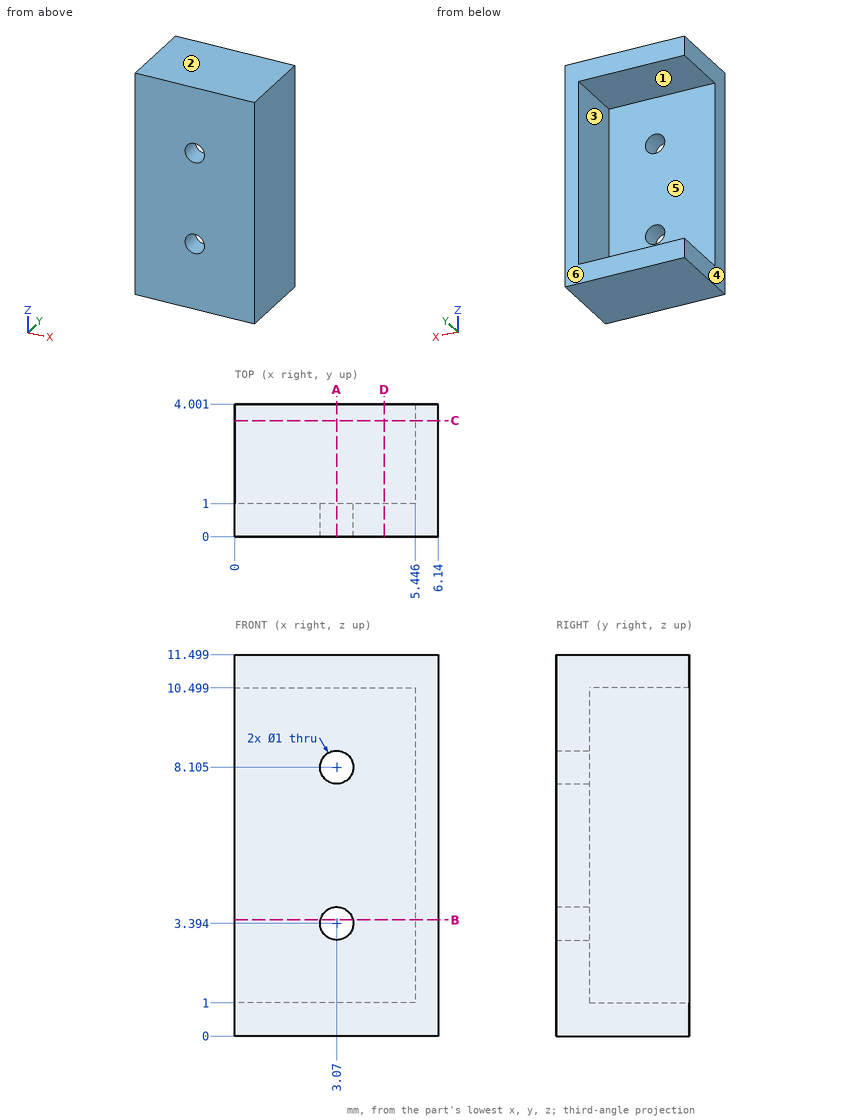
Geometry check sheet. Reference: drawing and pictorial views, mm from the part's lowest x, y, z. A direction names the side the tool comes from. Round coordinates to 2 decimals unless told otherwise and drop trailing zeros. Order: outer loops, then holes, each group sorted by start corner. A loop starts at its lowest first (then second) coordinate and runs counter-clockwise, first axis right, second up. Notation, with made-up numbers: (8, 63.25) -> (50, 63.25) arc R19 ccw to (50, 73.25) -> close; hole circle Ø7 at (41.25, -35.75). An arc over 180 degrees is marked (long way). One line per item, written item: value. Start each with the question number.
Q1. Cross-section at A-A (x = 3.07). Record the boundary of the cut face in (y, z) (1 decimal).
Q2. Gauge pin test, flat ends, axial feed: pin 1 Ø1.6 at (x, z) = (1.5, 8) entering from +Y; pin 2 Ø1.5 at (y, z) = (2.5, 6.5) entering from -X. Record the tip position at first contact, or that the pin passes through.
Q3. Thickness scan on line 1 (Z direction, x = 3.07, y = 0.6) (1 decimal); line 2 (Z direction, x = 3.5, y = 2); line 3 (X direction, y = 1.75, z = 4.75) (1 decimal). Record the ranges inside material, lowest first.
Q4. Cross-section at D-D (x = 4.5). Record the boundary of the cut face in (y, z).
Q5. Cross-section at C-C (y = 3.5). Record the boundary of the cut face in (x, z) (1 decimal).
Q6. Mould release check, pull along Z, two halves, no side actions. Record for the marked faces 1, 2, 3 and 4: pulls with the +Z half, pulls with the -Z half, needs draft (parallel to the pull), parting line crosses it, or undercut.
Q7. Set-up check for the marked faces 5 and 6: record each of +Z, -Z, +X, -X, +Y, -Y from which the full face is reachable in a straight line by a thin tool's end or side.
Q8. Cross-section at B-B (z = 3.5). Record the boundary of the cut face in (x, y) (1 decimal).
Completed:
1. outline: (0, 0) -> (4, 0) -> (4, 1) -> (1, 1) -> (1, 2.9) -> (0, 2.9) -> close; (0, 3.9) -> (1, 3.9) -> (1, 7.6) -> (0, 7.6) -> close; (0, 8.6) -> (1, 8.6) -> (1, 10.5) -> (4, 10.5) -> (4, 11.5) -> (0, 11.5) -> close
2. pin 1: stops at y = 1
2. pin 2: stops at x = 5.45
3. line 1: z = 0 to 2.9, 3.9 to 7.6, 8.6 to 11.5
3. line 2: z = 0 to 1, 10.5 to 11.5
3. line 3: x = 5.4 to 6.1
4. outline: (0, 0) -> (4, 0) -> (4, 1) -> (1, 1) -> (1, 10.5) -> (4, 10.5) -> (4, 11.5) -> (0, 11.5) -> close
5. outline: (0, 0) -> (6.1, 0) -> (6.1, 11.5) -> (0, 11.5) -> (0, 10.5) -> (5.4, 10.5) -> (5.4, 1) -> (0, 1) -> close
6. face 1: undercut
6. face 2: pulls with the +Z half
6. face 3: undercut
6. face 4: needs draft
7. face 5: -X, +Y
7. face 6: +Z, -Z, +X, -X, +Y
8. outline: (0, 0) -> (2.6, 0) -> (2.6, 1) -> (0, 1) -> close; (3.6, 0) -> (6.1, 0) -> (6.1, 4) -> (5.4, 4) -> (5.4, 1) -> (3.6, 1) -> close
